Work out the finished part from the listing and answer in its coordinate system (mm). Face numbers are marked on the shaded views. A direction names the side the tool comes from. Coordinates: 2 decimals unless noted, no trailing zeros. Write each loop counter-clockwise with the first axis right and the second up, starting at its lowest first coordinate (ties: lowest second). Pieces come first, ordered by that corner, then holes. Notation, with made-up numbers: (-5.75, -3) - (31.25, -3) arc R9 ccw to (31.25, 2) - close; hole circle Ø1 at (82.25, 35). An arc over 180 degrees is marked (long way). Use one line per item in the form item = value. Start each with the question number.
Item 1: A cutting plane is placed at A-A (x = 15.95). Write down the section's boundary in (y, z).
Item 2: Given pin 1 (19.5 mm diameter, centred on y = 0, z = 0, fed in from +X); pin 2 (2 mm diameter, centred on x = 85, z = -7.5, fed in from +Y); pin 3 (1.5 mm diameter, centred on x = 49.5, z = 33.5, fed in from -Y); pin 4 (4 mm diameter, centred on x = 154, y = -7, fed in from -Z), each flat-ended and moving along its own axis, determine where each tip first touches the part or whether it passes through.
Item 3: Consider probe 1 along Y at (x, z) = (32.5, 0); probe 2 along X at (y, z) = (-16, -3.5); probe 3 along Z at (x, y) = (144.5, 0). Determine where each line is inside the solid, lowest interval first.
Item 4: Determine the mould class of the marked faces 3, 4 and 5 for opening direction Y: released by +Y, released by -Y, zero draft, split by the parting line, or undercut.
Item 5: For the marked faces 1 and 2, determine the directions among +Z, -Z, +X, -X, +Y, -Y from which every point of the face is accessible in a straight line to the end or side of a thin tool.
from build123d import *

# Parameters (mm, degrees)
FILLET1_R          = 2
FILLET2_R          = 1
SKETCH5_R          = 2.2
CUT_EXTRUDE1_DEPTH = 212.443107005


with BuildPart() as part:
    # Sketch2 → Revolve1 (revolve)
    with BuildSketch(Plane(origin=(0, 0, 0), x_dir=(1, 0, 0), z_dir=(0, 1, 0))):
        with BuildLine():
            Line((8.8, -32.1), (12.1, -44.75))
            Line((12.1, -44.75), (63.8, -44.75))
            Line((63.8, -44.75), (68.2, -39.6))
            Line((68.2, -39.6), (68.2, -22))
            Line((68.2, -22), (201.75, -18.7))
            Line((201.75, -18.7), (201.75, -13.2))
            Line((201.75, -13.2), (157.75, -13.2))
            ThreePointArc((157.75, -13.2), (157.031986163, -12.818013837), (156.65, -12.1))
            Line((156.65, -12.1), (156.25, -12.1))
            Line((156.25, -12.1), (156.25, -13.2))
            Line((156.25, -13.2), (155.15, -13.2))
            Line((155.15, -13.2), (155.15, -12.1))
            Line((155.15, -12.1), (131.05, -12.1))
            Line((131.05, -12.1), (131.05, -12.65))
            Line((131.05, -12.65), (129.95, -12.65))
            Line((129.95, -12.65), (129.95, -10.45))
            Line((129.95, -10.45), (56.1, -10.45))
            Line((56.1, -10.45), (56.1, -26))
            Line((56.1, -26), (51.7, -26))
            Line((51.7, -26), (51.7, -31))
            Line((51.7, -31), (23.1, -31))
            Line((23.1, -31), (23.1, -32.1))
            Line((23.1, -32.1), (8.8, -32.1))
        make_face()
    revolve(axis=Axis((0, 0, 0), (1, 0, 0)))

    # Fillet1
    fillet1_edges = [part.edges().sort_by_distance(p)[0] for p in [
        (201.75, 0, -18.7),
    ]]
    fillet(fillet1_edges, radius=FILLET1_R)

    # Fillet2
    fillet2_edges = [part.edges().sort_by_distance(p)[0] for p in [
        (51.7, 0, -31),
    ]]
    fillet(fillet2_edges, radius=FILLET2_R)

    # Sketch5 → Cut-Extrude1 (cut, through all)
    with BuildSketch(Plane.XY):
        with Locations((15.95, 0)):
            Circle(SKETCH5_R)
    extrude(amount=-CUT_EXTRUDE1_DEPTH, mode=Mode.SUBTRACT)


solid = part.part
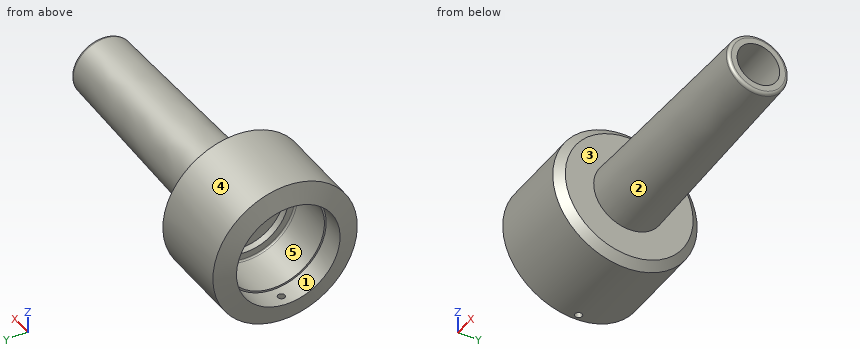
Answer:
q1.outline = (-2.2, -44.7) - (-2.2, -32.02) arc R32.1 cw (long way) to (2.2, -32.02) - (2.2, -44.7) arc R44.75 ccw (long way) to start
q2.pin_1 = through
q2.pin_2 = 20.58
q2.pin_3 = -30.5
q2.pin_4 = -19.24
q3.probe_1 = -44.75 to -31, 31 to 44.75
q3.probe_2 = 56.1 to 201.75
q3.probe_3 = -20.11 to -12.1, 12.1 to 20.11
q4.face_3 = zero draft
q4.face_4 = split by the parting line
q4.face_5 = undercut
q5.face_1 = -X
q5.face_2 = +X
